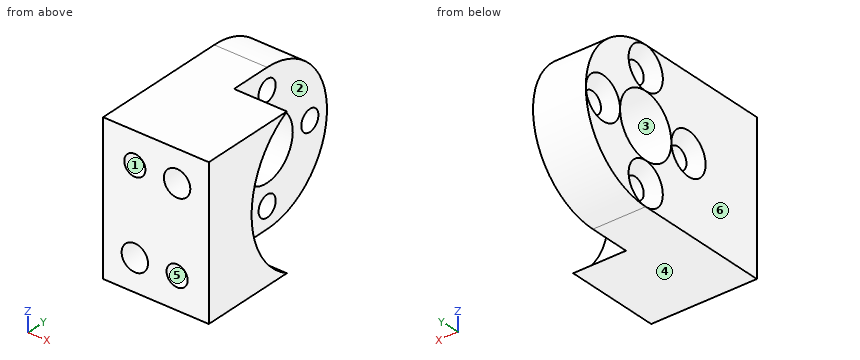
```python
from build123d import *

# Parameters (mm, degrees)
SKETCH1_R                       = 3
SKETCH1_R_2                     = 1
BOSS_EXTRUDE1_DEPTH             = 10
SKETCH2_R                       = 8
CUT_EXTRUDE1_DEPTH              = 5
CIRPATTERN1_OUTLINE_R           = 1
CIRPATTERN1_DEPTH               = 5
TAP_DRILL_FOR_M3X0_5_TAP1_D     = 2.5
TAP_DRILL_FOR_M3X0_5_TAP1_DEPTH = 4
TAP_DRILL_FOR_M3X0_5_TAP1_TIP   = 0.751075774
SKETCH5_R                       = 1
CUT_EXTRUDE2_DEPTH              = 4
CHAMFER1_SIZE                   = 1


# Read off the part's stored shape, not the designer's step: CirPattern1
with BuildPart() as part:
    # Sketch1 → Boss-Extrude1 (new body)
    with BuildSketch(Plane(origin=(0, 0, 0), x_dir=(0, 0, -1), z_dir=(1, 0, 0))):
        with BuildLine():
            Line((0, 13), (0, 0))
            Line((0, 0), (14, 0))
            Line((14, 0), (14, 13))
            ThreePointArc((14, 13), (7, 20), (0, 13))
        make_face()
        with Locations((7, 13)):
            Circle(SKETCH1_R, mode=Mode.SUBTRACT)
        with Locations((12, 13)):
            Circle(SKETCH1_R_2, mode=Mode.SUBTRACT)
    extrude(amount=BOSS_EXTRUDE1_DEPTH)

    # Sketch2 → Cut-Extrude1 (cut)
    with BuildSketch(Plane(origin=(10, 0, 0), x_dir=(0, 0, -1), z_dir=(1, 0, 0))):
        with Locations((7, 13)):
            Circle(SKETCH2_R)
    extrude(amount=-CUT_EXTRUDE1_DEPTH, mode=Mode.SUBTRACT)

    # CirPattern1 outline → CirPattern1 (cut)
    with BuildSketch(Plane.YZ):
        with Locations((8, -7)):
            Circle(CIRPATTERN1_OUTLINE_R)
        with Locations((13, -2)):
            Circle(CIRPATTERN1_OUTLINE_R)
        with Locations((18, -7)):
            Circle(CIRPATTERN1_OUTLINE_R)
    extrude(amount=CIRPATTERN1_DEPTH, mode=Mode.SUBTRACT)

    # Tap Drill for M3x0.5 Tap1
    with Locations(Plane(origin=(0, 0, 0), x_dir=(-1, 0, 0), z_dir=(0, -1, 0))):
        with Locations((-3, 11), (-7, 3)):
            Hole(TAP_DRILL_FOR_M3X0_5_TAP1_D / 2, depth=TAP_DRILL_FOR_M3X0_5_TAP1_DEPTH)
            with Locations((0, 0, -(TAP_DRILL_FOR_M3X0_5_TAP1_DEPTH + TAP_DRILL_FOR_M3X0_5_TAP1_TIP / 2))):  # 118° drill point
                Cone(0, TAP_DRILL_FOR_M3X0_5_TAP1_D / 2, TAP_DRILL_FOR_M3X0_5_TAP1_TIP, mode=Mode.SUBTRACT)

    # Sketch5 → Cut-Extrude2 (cut)
    with BuildSketch(Plane.XZ):
        with Locations(Location((3, -3, 0), (0, 0, 270))):
            Circle(SKETCH5_R)
        with Locations(Location((7, -11, 0), (0, 0, 270))):
            Circle(SKETCH5_R)
    extrude(amount=-CUT_EXTRUDE2_DEPTH, mode=Mode.SUBTRACT)

    # Chamfer1
    chamfer1_edges = [part.edges().sort_by_distance(p)[0] for p in [
        (0, 13, -11),
        (0, 17, -7),
        (0, 12, -2),
        (0, 7, -7),
    ]]
    chamfer(chamfer1_edges, length=CHAMFER1_SIZE - 0.0001)  # a hair under: the kernel refuses the full size


solid = part.part
```
Here's how the part is built. I have some questions about the finished solid (model axes, mm). Face numbers are marked on the shaded views. A direction names the side the tool comes from. Coordinates: 2 decimals unless noted, no trailing zeros. Order: outer loops, then holes, each group sorted by start corner. A loop starts at its lowest first (then second) coordinate and runs counter-clockwise, first axis right, second up.
1) Imagine slicing it at B-B on x = 4.5. List the corners of the cut face in (y, z) for me.
2) Will these pins go through, and if not, where does the flat tip stop? pin 1 (4 mm diameter, centred on y = 10.5, z = -7.5, fed in from +X); pin 2 (2 mm diameter, centred on x = 8, z = -9, fed in from +Y); pin 3 (1.2 mm diameter, centred on x = 7, z = -11, fed in from -Y).
3) I need wall thicknesses on line 1 (X direction, y = 14.25, z = -10); line 2 (X direction, y = 2.25, z = -11.25); line 3 (Z direction, x = 3, y = 13.25). Which ranges of each line are inside material? Lowest first, please.
4) Imagine slicing it at D-D on y = 5.5. List the corners of the cut face in (x, z) for me, and give its area (3 significant figures).
5) Which directions (+Z, -Z, +X, -X, +Y, -Y) give clear straight access to the entire face, cutting with the end or side of a thin tool? Please do the marked faces 1, 2 and 3.
6) We'd pull the mould along Z, two halves only. Please class the marked faces 4, 5 and 6: +Z half, -Z half, draft (parallel to the pull), parting line (faces both ways), or undercut.
7) Imagine slicing it at A-A on y = 3. List the corners of the cut face in (x, z) for me.
8) Imagine slicing it at C-C on y = 10.75. List the corners of the cut face in (x, z) for me.
Response values:
1. outline: (0, -14) - (13, -14) arc R7 ccw to (13, 0) - (0, 0) - close; hole circle Ø2 at (8, -7); hole circle Ø6 at (13, -7); hole circle Ø2 at (13, -12); hole circle Ø2 at (13, -2); hole circle Ø2 at (18, -7)
2. pin 1: stops at x = 5
2. pin 2: stops at y = 5.58
2. pin 3: stops at y = 4
3. line 1: x = 0 to 5
3. line 2: x = 0 to 1.78, 4.22 to 6.03, 7.97 to 10
3. line 3: z = -14 to -12.97, -11.03 to -9.99, -4.01 to -2.97, -1.03 to 0
4. outline: (0, -14) - (10, -14) - (10, -9.78) - (5, -9.78) - (5, -4.22) - (10, -4.22) - (10, 0) - (0, 0) - close
4. area: 112 mm2
5. face 1: -Y
5. face 2: +X, +Y
5. face 3: +X, -X
6. face 4: -Z half
6. face 5: undercut
6. face 6: draft
7. outline: (0, -14) - (10, -14) - (10, 0) - (0, 0) - close; hole circle Ø2.5 at (3, -11); hole circle Ø2 at (3, -3); hole circle Ø2.5 at (7, -3); hole circle Ø2 at (7, -11)
8. outline: (0, -14) - (5, -14) - (5, -8.98) - (0, -8.98) - close; (0, -5.02) - (5, -5.02) - (5, 0) - (0, 0) - close
